```python
from build123d import *

# Parameters (mm, degrees)
PAD001_DEPTH    = 55
FILLET002_R     = 5
SKETCH006_R     = 2
POCKET001_DEPTH = 55.001
POCKET002_START = 30
POCKET002_DEPTH = 70


with BuildPart() as part:
    # Sketch001 → Pad001 (new body)
    with BuildSketch(Plane.XY):
        with BuildLine():
            Line((0, 0), (-22.231309, 61.08002))
            Line((-22.231309, 61.08002), (3.869698, 61.08002))
            Line((3.869698, 61.08002), (20.319194, 37.587705))
            Line((20.319194, 37.587705), (26.673169, 20.130302))
            ThreePointArc((12.57778, 0), (24.865061, 6.396353), (26.673169, 20.130302))
            Line((12.57778, 0), (0, 0))
        make_face()
    extrude(amount=PAD001_DEPTH)

    # Fillet002
    fillet002_edges = [part.edges().sort_by_distance(p)[0] for p in [
        (20.319194, 37.587705, 27.5),
        (0, 0, 27.5),
        (3.869698, 61.08002, 27.5),
        (-22.231309, 61.08002, 27.5),
        (-11.115655, 30.54001, 55),
        (-9.180806, 61.08002, 55),
        (12.094446, 49.333863, 55),
        (23.496182, 28.859003, 55),
        (24.865061, 6.396353, 55),
        (6.28889, 0, 55),
    ]]
    fillet(fillet002_edges, radius=FILLET002_R)

    # Sketch006 → Pocket001 (cut, through all)
    with BuildSketch(Plane.XY):
        with Locations((12, 12)):
            Circle(SKETCH006_R)
        with Locations((-6, 50)):
            Circle(SKETCH006_R)
    extrude(amount=POCKET001_DEPTH, mode=Mode.SUBTRACT)

    # Sketch007 → Pocket002 (cut)
    with BuildSketch(Plane.XY.offset(POCKET002_START)):
        Polygon((14.078461, 15.6), (9.921539, 15.6), (7.843078, 12), (9.921539, 8.4), (14.078461, 8.4), (16.156922, 12), align=None)
        Polygon((-1.843078, 50), (-3.921539, 53.6), (-8.078461, 53.6), (-10.156922, 50), (-8.078461, 46.4), (-3.921539, 46.4), align=None)
    extrude(amount=POCKET002_DEPTH, mode=Mode.SUBTRACT)


solid = part.part
```
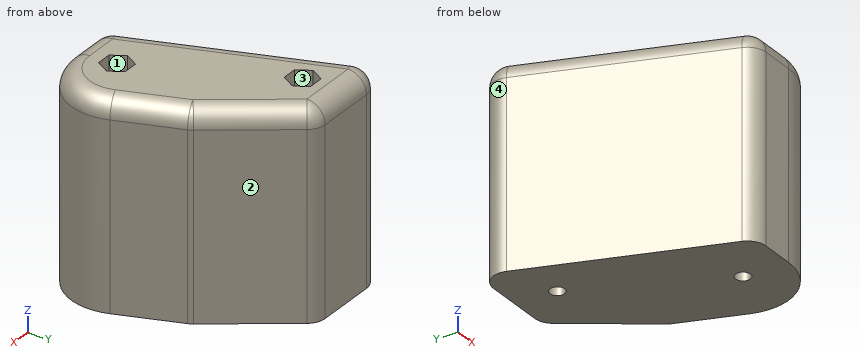
CAD build for the part. Positions are in the model's coordinates, mm. Face numbers are marked on the shaded views. Round coordinates to 2 decimals unless told otherwise and drop trailing zeros. Order: outer loops, then holes, each group sorted by start corner. A loop starts at its lowest first (then second) coordinate and runs counter-clockwise, first axis right, second up. Notation, with made-up numbers: (81, -8) -> (114, -8) arc R24 ccw to (114, 30) -> close; hole circle Ø9 at (22, 87.25). An arc over 180 degrees is marked (long way). Write item = value, one per line.
(1) Flat gauge pins, fed straight in: P1, Ø5, axis at y = 20.5, z = 26.5, coming from the -X side; P2, Ø8, axis at x = 1, y = 42.5, coming from the -Z side; P3, Ø12, axis at x = 8.5, z = 29.5, coming from the +Y side; P4, Ø3, axis at x = 13, z = 41.5, coming from the +Y side. Where does each tip first touch, or does it go through?
Answers follow:
P1 = -8.37
P2 = 0
P3 = 60.93
P4 = 50.18
(2) Cut at A-A (z = 42). Write the cut outline in (x, y).
Answers follow:
outline = (-19.79, 54.37) -> (-1.2, 3.29) arc R5 ccw to (3.5, 0) -> (12.58, 0) arc R15 ccw to (26.67, 20.13) -> (20.54, 36.97) arc R5 ccw to (19.94, 38.13) -> (5.36, 58.95) arc R5 ccw to (1.27, 61.08) -> (-15.09, 61.08) arc R5 ccw to start; hole (-10.16, 50) -> (-8.08, 46.4) -> (-3.92, 46.4) -> (-1.84, 50) -> (-3.92, 53.6) -> (-8.08, 53.6) -> close; hole (7.84, 12) -> (9.92, 8.4) -> (14.08, 8.4) -> (16.16, 12) -> (14.08, 15.6) -> (9.92, 15.6) -> close
(3) Cut at B-B (z = 28.5). Write the cut outline in (x, y).
Answers follow:
outline = (-19.79, 54.37) -> (-1.2, 3.29) arc R5 ccw to (3.5, 0) -> (12.58, 0) arc R15 ccw to (26.67, 20.13) -> (20.54, 36.97) arc R5 ccw to (19.94, 38.13) -> (5.36, 58.95) arc R5 ccw to (1.27, 61.08) -> (-15.09, 61.08) arc R5 ccw to start; hole circle Ø4 at (-6, 50); hole circle Ø4 at (12, 12)
(4) Drill centre lines: L1, parallel to X at y = 13.5, z = 6.5; L2, parallel to X at y = 50, z = 8; L3, parallel to Z at x = 12, y = 9. Where is each one in solid material? Low to high.
Answers follow:
L1 = -4.91 to 10.68, 13.32 to 27.5
L2 = -18.2 to -8, -4 to 11.63
L3 = 0 to 30
(5) Cut at C-C (z = 52). Write the cut outline in (x, y), plus the area to 3 significant figures.
Answers follow:
outline = (-19.4, 54.51) -> (-0.81, 3.43) arc R4.58 ccw to (3.5, 0.42) -> (12.58, 0.42) arc R14.58 ccw to (26.28, 19.99) -> (20.15, 36.83) arc R4.58 ccw to (19.6, 37.89) -> (5.02, 58.71) arc R4.58 ccw to (1.27, 60.66) -> (-15.09, 60.66) arc R4.58 ccw to start; hole (-10.16, 50) -> (-8.08, 46.4) -> (-3.92, 46.4) -> (-1.84, 50) -> (-3.92, 53.6) -> (-8.08, 53.6) -> close; hole (7.84, 12) -> (9.92, 8.4) -> (14.08, 8.4) -> (16.16, 12) -> (14.08, 15.6) -> (9.92, 15.6) -> close
area = 1,700 mm²
(6) Pull direction Y, two halves, no side cores. Call the marked faces 1, 2, 3 and 4: +Y half, -Y half, draft (parallel to the pull), parting line (faces both ways), or undercut.
Answers follow:
face_1 = undercut
face_2 = +Y half
face_3 = undercut
face_4 = parting line
